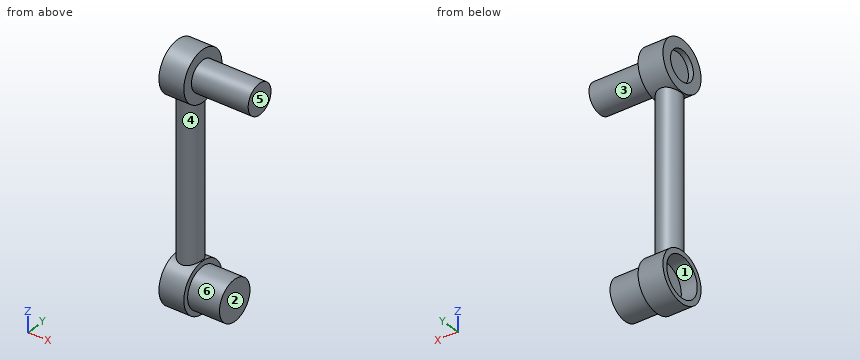
from build123d import *

# Parameters (mm, degrees)
SKETCH1_R           = 29.21
BOSS_EXTRUDE1_DEPTH = 406.4
SKETCH2_W           = 63.5
SKETCH2_H           = 63.5
SKETCH3_R           = 50.8
BOSS_EXTRUDE2_DEPTH = 81.28
SKETCH10_W          = 63.5
SKETCH10_H          = 63.5
SKETCH5_R           = 50.8
CUT_EXTRUDE1_DEPTH  = 40.64
SKETCH11_R          = 38.1
BOSS_EXTRUDE4_DEPTH = 144.78
SKETCH16_R          = 38.1
CUT_EXTRUDE2_DEPTH  = 12.7
SCALE1_SCALE        = 0.03937


with BuildPart() as part:
    # Sketch1 → Boss-Extrude1 (new body)
    with BuildSketch(Plane.XY):
        Circle(SKETCH1_R)
    extrude(amount=BOSS_EXTRUDE1_DEPTH)

    # Sketch2 → Revolve1 (revolve)
    with BuildSketch(Plane(origin=(0, 0, 0), x_dir=(1, 0, 0), z_dir=(0, 1, 0))):
        with Locations((0, 19.05)):
            Rectangle(SKETCH2_W, SKETCH2_H)
    revolve(axis=Axis((-31.75, 0, -50.8), (1, 0, 0)))

    # Sketch3 → Boss-Extrude2 (add)
    with BuildSketch(Plane(origin=(31.75, 0, 0), x_dir=(0, 0, -1), z_dir=(1, 0, 0))):
        with Locations((50.8, 0)):
            Circle(SKETCH3_R)
    extrude(amount=BOSS_EXTRUDE2_DEPTH)

    # Sketch10 → Revolve2 (revolve)
    with BuildSketch(Plane(origin=(0, 0, 0), x_dir=(1, 0, 0), z_dir=(0, 1, 0)), mode=Mode.PRIVATE) as revolve2_sk:
        with Locations((0, -425.45)):
            Rectangle(SKETCH10_W, SKETCH10_H)
    revolve(revolve2_sk.sketch.rotate(Axis((-31.75, 0, 457.2), (1, 0, 0)), 180), axis=Axis((-31.75, 0, 457.2), (1, 0, 0)))

    # Sketch5 → Cut-Extrude1 (cut)
    with BuildSketch(Plane.ZY.offset(31.75)):
        with Locations(Location((-50.8, 0, 0), (0, 0, 180))):
            Circle(SKETCH5_R)
    extrude(amount=-CUT_EXTRUDE1_DEPTH, mode=Mode.SUBTRACT)

    # Sketch11 → Boss-Extrude4 (add)
    with BuildSketch(Plane(origin=(31.75, 0, 0), x_dir=(0, 0, -1), z_dir=(1, 0, 0))):
        with Locations((-457.2, 0)):
            Circle(SKETCH11_R)
    extrude(amount=BOSS_EXTRUDE4_DEPTH)

    # Sketch16 → Cut-Extrude2 (cut)
    with BuildSketch(Plane.ZY.offset(31.75)):
        with Locations(Location((457.2, 0, 0), (0, 0, 180))):
            Circle(SKETCH16_R)
    extrude(amount=-CUT_EXTRUDE2_DEPTH, mode=Mode.SUBTRACT)


with BuildPart() as part_1:
    # Scale1: scaled about (34.078233281, 5.4627e-05, 222.606303222)
    add(part.part.scale(SCALE1_SCALE).moved(Location((32.736573237, 5.2476e-05, 213.842293064))))


solid = part_1.part
The model under review builds one solid part; all positions refer to its coordinate system, in mm. Face numbers are marked on the shaded views. A direction names the side the tool comes from. Give positions to 0.01 mm unless a question says otherwise; leave off trailing zeros. Loops run counter-clockwise (first coordinate to the right, second up) from the corner with the lowest first, then second, coordinate; pieces in that order, holes last. Notation, with made-up numbers: (9, 5) -> (25, 5) arc R12 cw to (25, 20) -> close; hole circle Ø1 at (42.25, 57). An arc over 180 degrees is marked (long way). Put each result on its own line as item: value. Start each with the question number.
1. For the marked faces 1, 2 and 3, list the 3-axis set-ups (+Z, -Z, +X, -X, +Y, -Y) from which the entire face can be reached by the end or side of a thin tool; tool diameter is ignored.
2. Wall thickness on probe 1 along Z at (x, y) = (36, 0); probe 2 along X at (y, z) = (1.4, 230.75); probe 3 along Z at (x, y) = (32.5, 0.7): over which ranges is each line inside the solid? List them lowest first.
3. We need section A-A on y = -0.4. State the section outline as (x, z) points.
4. We need section D-D on x = 32.75. State the section outline as (y, z) points.
5. We need section B-B on x = 35.25. State the section outline as (y, z) points.
6. Clearance check with flat-ended pins moving along their axes: P1, Ø2, axis at y = 0, z = 212.5, coming from the +X side; P2, Ø1.5, axis at y = 0.5, z = 219, coming from the -X side; P3, Ø2, axis at y = -1.5, z = 217.5, coming from the -X side. State where each tip first meets the part, or that it passes through.
7. We need section C-C on z = 211. State the section outline as (x, y) points, then the cut area to 3 significant figures.
8. Mouldability with a two-part tool opening along X and no side actions: class the marked faces 4, 5 and 6 as released by +X, released by -X, zero draft, split by the parting line, or undercut.
Determined:
1. face 1: -X
1. face 2: -Z, +X, +Y, -Y
1. face 3: +X
2. probe 1: 209.84 to 213.84, 230.34 to 233.34
2. probe 2: 31.49 to 33.99
2. probe 3: 209.44 to 209.97, 213.72 to 234.24
3. outline: (31.49, 209.37) -> (33.99, 209.37) -> (33.99, 209.88) -> (37.19, 209.88) -> (37.19, 213.8) -> (33.99, 213.8) -> (33.99, 214.31) -> (33.81, 214.31) -> (33.81, 229.37) -> (33.99, 229.37) -> (33.99, 230.4) -> (39.69, 230.4) -> (39.69, 233.29) -> (33.99, 233.29) -> (33.99, 234.31) -> (31.49, 234.31) -> (31.49, 233.29) -> (31.99, 233.29) -> (31.99, 230.4) -> (31.49, 230.4) -> (31.49, 229.37) -> (31.66, 229.37) -> (31.66, 214.31) -> (31.49, 214.31) -> (31.49, 213.8) -> (33.09, 213.8) -> (33.09, 209.88) -> (31.49, 209.88) -> close
4. outline: (-1.15, 214.06) arc R2.5 ccw (long way) to (1.15, 214.06) -> (1.15, 229.62) arc R2.5 ccw (long way) to (-1.15, 229.62) -> close; hole circle Ø4 at (0, 211.84)
5. outline: circle Ø4 at (0, 211.84); circle Ø3 at (0, 231.84)
6. P1: x = 37.19
6. P2: x = 31.59
6. P3: x = 31.7
7. outline: (31.49, -2.35) -> (33.99, -2.35) -> (33.99, -1.81) -> (37.19, -1.81) -> (37.19, 1.81) -> (33.99, 1.81) -> (33.99, 2.35) -> (31.49, 2.35) -> (31.49, 1.81) -> (33.09, 1.81) -> (33.09, -1.81) -> (31.49, -1.81) -> close
7. area: 17.6 mm^2
8. face 4: split by the parting line
8. face 5: released by +X
8. face 6: zero draft
